from build123d import *

# Parameters (mm, degrees)
SKETCH1_R                  = 10.5
BOSS_EXTRUDE1_DEPTH        = 18
SKETCH3_R                  = 0.487346303
BOSS_EXTRUDE2_DEPTH        = 0.8
M5_TAPPED_HOLE1_AT_2_COUNT = 2
M5_TAPPED_HOLE1_AT_2_PITCH = 26
M5_TAPPED_HOLE1_AT_3_COUNT = 2
M5_TAPPED_HOLE1_AT_3_PITCH = 30.5
M5_TAPPED_HOLE1_AT_4_COUNT = 2
M5_TAPPED_HOLE1_AT_4_PITCH = 40.078048855
CHAMFER1_SIZE              = 0.2
CHAMFER1_SIZE2             = 0.346410162
CHAMFER1_PART_2_SIZE       = 0.2
CHAMFER1_PART_2_SIZE2      = 0.346410162


with BuildPart() as part:
    # Sketch1 → Boss-Extrude1 (new body, symmetric)
    with BuildSketch(Plane.XY):
        Polygon((-9, -1), (9, -1), (11, 0), (21, 0), (21, -8), (19.5, -12), (19.5, -24), (11, -24), (7.5, -28), (-7.5, -28), (-11, -24), (-19.5, -24), (-19.5, -12), (-21, -8), (-21, 0), (-11, 0), align=None)
        with Locations((0, -15)):
            Circle(SKETCH1_R, mode=Mode.SUBTRACT)
    extrude(amount=BOSS_EXTRUDE1_DEPTH, both=True)

    # Sketch2 → Revolve1 (revolve)
    with BuildSketch(Plane(origin=(0, 0, 0), x_dir=(0, 0, -1), z_dir=(1, 0, 0))):
        Polygon((-15, -4.5), (15, -4.5), (15, -5.6), (14.2, -5.6), (14.2, -8.2), (14.8, -8.2), (14.8, -9), (-14.8, -9), (-14.8, -8.2), (-14.2, -8.2), (-14.2, -5.6), (-15, -5.6), align=None)
    revolve(axis=Axis((0, -15, 30.2753079), (0, 0, -1)))

    # Sketch3 → Boss-Extrude2 (add)
    with BuildSketch(Plane.XY.offset(15)):
        with BuildLine():
            Line((1.141194716, -4.059356755), (0.643070986, -5.356749026))
            ThreePointArc((0.643070986, -5.356749026), (1.151535438, -6.713388037), (2.559436926, -6.371600228))
            ThreePointArc((2.559436926, -6.371600228), (0, -24), (-2.559436926, -6.371600228))
            ThreePointArc((-2.559436926, -6.371600228), (-1.151535438, -6.713388037), (-0.643070986, -5.356749026))
            Line((-0.643070986, -5.356749026), (-1.141194716, -4.059356755))
            ThreePointArc((-1.141194716, -4.059356755), (0, -26), (1.141194716, -4.059356755))
        make_face()
        with Locations((1.662663475, -5.748213677)):
            Circle(SKETCH3_R, mode=Mode.SUBTRACT)
        with Locations((-1.662663475, -5.748213677)):
            Circle(SKETCH3_R, mode=Mode.SUBTRACT)
    boss_extrude2 = extrude(amount=BOSS_EXTRUDE2_DEPTH)

    # Mirror1: Boss-Extrude2 across plane
    add(boss_extrude2.mirror(Plane.XY))

    # Sketch6 → M5 Tapped Hole1 (revolve, cut)
    with BuildSketch(Plane(origin=(15.25, 0, -13), x_dir=(0, 0, 1), z_dir=(1, 0, 0))):
        Polygon((0, 0), (0, 24), (2.5, 24), (2.1, 23.6), (2.1, 12), (2.5, 12), (2.5, 0), align=None)
    m5_tapped_hole1 = revolve(axis=Axis((15.25, 6.35, -13), (0, -1, 0)), mode=Mode.SUBTRACT)

    # M5 Tapped Hole1 at 2: M5 Tapped Hole1 ×2
    with Locations(*[(0, 0, i * M5_TAPPED_HOLE1_AT_2_PITCH) for i in range(1, M5_TAPPED_HOLE1_AT_2_COUNT)]):
        add(m5_tapped_hole1, mode=Mode.SUBTRACT)

    # M5 Tapped Hole1 at 3: M5 Tapped Hole1 ×2
    with Locations(*[(-i * M5_TAPPED_HOLE1_AT_3_PITCH, 0, 0) for i in range(1, M5_TAPPED_HOLE1_AT_3_COUNT)]):
        add(m5_tapped_hole1, mode=Mode.SUBTRACT)

    # M5 Tapped Hole1 at 4: M5 Tapped Hole1 ×2
    with Locations(*[Vector(-0.761015091, 0, 0.648734176) * (i * M5_TAPPED_HOLE1_AT_4_PITCH) for i in range(1, M5_TAPPED_HOLE1_AT_4_COUNT)]):
        add(m5_tapped_hole1, mode=Mode.SUBTRACT)

    # Chamfer1
    chamfer1_edges = [part.edges().sort_by_distance(p)[0] for p in [
        (-10.5, -15, -18),
    ]]
    chamfer1_side = [part.faces().sort_by_distance(p)[0] for p in [
        (-10.5, -15, -16.5),
    ]]
    chamfer(chamfer1_edges, length=CHAMFER1_SIZE, length2=CHAMFER1_SIZE2, reference=chamfer1_side[0])

    # Chamfer1 part 2
    chamfer1_part_2_edges = [part.edges().sort_by_distance(p)[0] for p in [
        (-10.5, -15, 18),
    ]]
    chamfer1_part_2_side = [part.faces().sort_by_distance(p)[0] for p in [
        (0, -1.504777179, 18),
    ]]
    chamfer(chamfer1_part_2_edges, length=CHAMFER1_PART_2_SIZE, length2=CHAMFER1_PART_2_SIZE2, reference=chamfer1_part_2_side[0])


solid = part.part
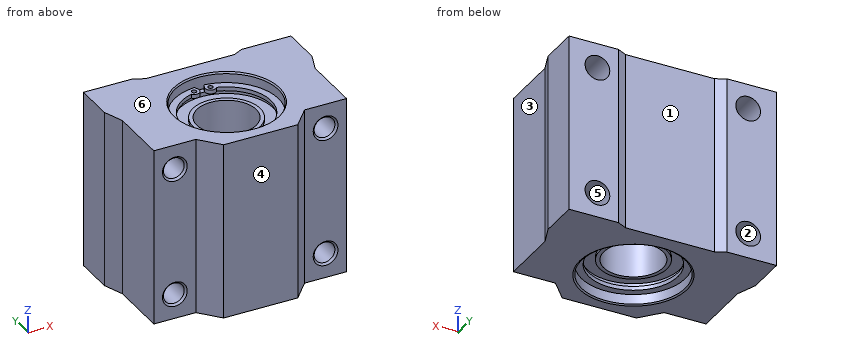
Design review of the part built by this model. Coordinates are the model's own, in mm. Face numbers are marked on the shaded views. A direction names the side the tool comes from. Round coordinates to 2 decimals unless told otherwise and drop trailing zeros. Write each loop counter-clockwise with the first axis right and the second up, starting at its lowest first coordinate (ties: lowest second). Pieces come first, ordered by that corner, then holes.
Item 1: For the marked faces 1, 2 and 3, list the 3-axis set-ups (+Z, -Z, +X, -X, +Y, -Y) from which the entire face can be reached by the end or side of a thin tool; tool diameter is ignored.
Item 2: Consider section C-C on z = -13. Count the separate pieces of the cut face and the enclosed holes in it, and give its area (3 significant figures).
Item 3: For pin 1 Ø14 at (x, y) = (0, -15) entering from -Z; pin 2 Ø5.5 at (x, z) = (-15.25, 13) entering from -Y; pin 3 Ø1.5 at (x, z) = (15.5, -12) entering from +Y; pin 4 Ø2 at (y, z) = (-17.5, -1) entering from +X, all flat-tipped, find the tip position at first contact; note any pin that passes through.
Item 4: Consider section B-B on x = -15.25. Give the boundary of the cut face in (y, z), and give its area (3 significant figures).
Item 5: Wall thickness on L1, parallel to X at y = -5, z = 13; L2, parallel to Y at x = 0, z = -15.5; L3, parallel to Z at x = -17, y = -6.5: over which ranges is each line inside the solid? List them lowest first.
Item 6: Draft analysis for pull direction Z (two halves, no side actions). For the marked faces 4, 5 and 6, state which applies: released by +Z, released by -Z, zero draft, split by the parting line, or undercut.
Item 7: Consider section A-A on z = -5. Give the boundary of the cut face in (x, y).
Check values:
1. face 1: +Z, -Z, +Y
1. face 2: +Y
1. face 3: +Z, -Z, +X, -Y
2. separate pieces: 3
2. enclosed holes: 1
2. area: 686 mm2
3. pin 1: stops at z = -14.8
3. pin 2: stops at y = -24
3. pin 3: passes through
3. pin 4: stops at x = 19.5
4. outline: (-24, -18) - (0, -18) - (0, -15.5) - (-12, -15.5) - (-12, -15.1) - (-23.6, -15.1) - (-24, -15.5) - close; (-24, -10.5) - (-23.6, -10.9) - (-12, -10.9) - (-12, -10.5) - (0, -10.5) - (0, 10.5) - (-12, 10.5) - (-12, 10.9) - (-23.6, 10.9) - (-24, 10.5) - close; (-24, 15.5) - (-23.6, 15.1) - (-12, 15.1) - (-12, 15.5) - (0, 15.5) - (0, 18) - (-24, 18) - close
4. area: 643 mm2
5. L1: x = -21 to -17.75, -12.75 to 12.75, 17.75 to 21
5. L2: y = -28 to -24, -4.5 to -1
5. L3: z = -18 to -14.79, -11.21 to 11.21, 14.79 to 18
6. face 4: zero draft
6. face 5: undercut
6. face 6: released by +Z
7. outline: (-21, -8) - (-19.5, -12) - (-19.5, -24) - (-11, -24) - (-7.5, -28) - (7.5, -28) - (11, -24) - (19.5, -24) - (19.5, -12) - (21, -8) - (21, 0) - (11, 0) - (9, -1) - (-9, -1) - (-11, 0) - (-21, 0) - close; hole circle Ø12 at (0, -15)
